from build123d import *

# Parameters (mm, degrees)
F2_R     = 4
F3_DEPTH = 70.001
F4_R     = 5


with BuildPart() as f1:
    # F0 (on Front) → F1 (revolve)
    with BuildSketch(Plane.XZ):
        Polygon((-45, 0), (0, 0), (0, 70), (-31.926143, 70), (-15.821369, 47), (-15.821369, 38), (-29.551464, 9), (-41.551464, 9), (-41.551464, 18), (-51.551464, 18), align=None)
    revolve(axis=Axis((0, 0, 35), (0, 0, 1)))

    # F2 (on face) → F3 (cut, through all)
    with BuildSketch(Plane(origin=(0, 0, 0), x_dir=(1, 0, 0), z_dir=(0, 0, -1))):
        with Locations((-36, 0)):
            Circle(F2_R)
        with Locations((-25.455844, -25.455844)):
            Circle(F2_R)
        with Locations((0, -36)):
            Circle(F2_R)
        with Locations((25.455844, -25.455844)):
            Circle(F2_R)
        with Locations((36, 0)):
            Circle(F2_R)
        with Locations((25.455844, 25.455844)):
            Circle(F2_R)
        with Locations((0, 36)):
            Circle(F2_R)
        with Locations((-25.455844, 25.455844)):
            Circle(F2_R)
    extrude(amount=-F3_DEPTH, mode=Mode.SUBTRACT)

    # F4
    f4_edges = [f1.edges().sort_by_distance(p)[0] for p in [
        (31.926143, 0, 70),
        (51.551464, 0, 18),
        (15.821369, 0, 47),
        (15.821369, 0, 38),
        (29.551464, 0, 9),
    ]]
    fillet(f4_edges, radius=F4_R)


solid = f1.part
Input: part model. Units: mm. Frame: model coordinates. A direction names the side the tool comes from. Give positions to 0.01 mm unless a question says otherwise; leave off trailing zeros. Write each loop counter-clockwise with the first axis right and the second up, starting at its lowest first coordinate (ties: lowest second). Pieces come first, ordered by that corner, then holes.
Q1. Set-up query: faces 5 (the face through (26, 33, 18)), 6 (the face through (-17.525, -5.519, 32.61)), 7 (the face through (32.8, 2.4, 4.4)). Return all of +Z, -Z, +X, -X, +Y, -Y with unobstructed straight access to the full face (end or side cutting, diameter ignored); none if empty.
Q2. Section B-B, the plane z = 42.5. Output: boundary loops of the cut face in (x, y).
Q3. First-contact query: P1, Ø13, axis at x = 25.46, y = 25.46, coming from the +Z side; P2, Ø10, axis at x = 29.5, y = -19.5, coming from the +Z side; P3, Ø6, axis at y = 6, z = 23, coming from the +X side. Flat tips, straight axial feed; report the tip coordinate or a pass-through.
Q4. Pull-direction query (Z, two-part tool) for faces 1 (the face through (0, 0, 70)), 2 (the face through (-14.6, 6.1, 42.2)), 3 (the face through (-15.88, 6.59, 48.96)), 4 (the face through (-0.521, -39.966, 4.437)); classes: pulls with the +Z half, pulls with the -Z half, needs draft (parallel to the pull), parting line crosses it, or undercut.
Q5. Material intervals for probe 1 along X at (y, z) = (14, 14.5); probe 2 along X at (y, z) = (0, 3.5); probe 3 along Z at (x, y) = (9.5, 17), sorted ascending.
Q6. Section A-A, the plane x = 0. State how many separate pieces and enclosed holes the cut face has, plus the area to 3 significant figures.
Q7. Section C-C, the plane z = 24. Output: boundary loops of the cut face in (x, y).
Filled in:
1. face 5: +Z
1. face 6: none
1. face 7: +Z, -Z
2. outline: circle Ø31.64 at (0, 0)
3. P1: stops at z = 18
3. P2: stops at z = 9.59
3. P3: stops at x = 23.74
4. face 1: pulls with the +Z half
4. face 2: undercut
4. face 3: undercut
4. face 4: needs draft
5. probe 1: x = -47.15 to -39.12, -23.03 to 23.03, 39.12 to 47.15
5. probe 2: x = -46.27 to -40, -32 to 32, 40 to 46.27
5. probe 3: z = 0 to 30.28, 52.22 to 70
6. separate pieces: 3
6. enclosed holes: 0
6. area: 3,480 mm2
7. outline: circle Ø44.9 at (0, 0)
